Design review of the part built by this model. Coordinates are the model's own, in mm. A direction names the side the tool comes from. Round coordinates to 2 decimals unless told otherwise and drop trailing zeros. Answer as CSV lines item,"result". Start each with the question number.
(1) For faces 5 (the flat face through (10, 2.5, 27)), 6 (the cylindrical face through (-46.91, 1.52, 23.8)), list the 3-axis set-ups (+Z, -Z, +X, -X, +Y, -Y) from which the entire face can be reached by the end or side of a thin tool; tool diameter is ignored.
(2) Wall thickness on L1, parallel to Y at x = 27.5, z = -1.5: over which ranges is the line inside the solid? List them lowest first.
(3) For P1, Ø4, axis at x = 19.5, z = -27.5, coming from the +Y side, flat-tipped, find the tip position at first contact; note if it passes through.
(4) Mouldability with a two-part tool opening along X and no side actions: class faces 1 (the flat face through (20, 0, -2)), 2 (the flat face through (-54.385, 1, -1)), 3 (the flat face through (23, 2.5, -28)), 4 (the flat face through (37, 2.5, -3)) as released by +X, released by -X, zero draft, split by the parting line, or undercut.
from build123d import *

# Parameters (mm, degrees)
SKETCH1_W           = 150
SKETCH1_H           = 60
BOSS_EXTRUDE1_DEPTH = 3
CUT_EXTRUDE1_REACH  = 102.604
SKETCH2_R           = 1.75
CUT_EXTRUDE2_DEPTH  = 0.5


with BuildPart() as part:
    # Sketch1 → Boss-Extrude1 (new body)
    with BuildSketch(Plane(origin=(0, 0, 0), x_dir=(1, 0, 0), z_dir=(0, 1, 0))):
        with Locations((20.614523463, 1.144067797)):
            Rectangle(SKETCH1_W, SKETCH1_H)
    extrude(amount=BOSS_EXTRUDE1_DEPTH)

    # Sketch2 → Cut-Extrude1 (cut, up to next)
    with BuildSketch(Plane(origin=(0, 3, 0), x_dir=(1, 0, 0), z_dir=(0, 1, 0)), mode=Mode.PRIVATE) as cut_extrude1_sk1:
        with Locations(Location((-48.385476537, 25.144067797, 0), (0, 0, 270))):
            Circle(SKETCH2_R)
    cut_extrude1_tool1 = extrude(cut_extrude1_sk1.sketch, amount=-CUT_EXTRUDE1_REACH, mode=Mode.PRIVATE) & part.part
    # Sketch2 → Cut-Extrude1 (cut, up to next)
    with BuildSketch(Plane(origin=(0, 3, 0), x_dir=(1, 0, 0), z_dir=(0, 1, 0)), mode=Mode.PRIVATE) as cut_extrude1_sk2:
        with Locations(Location((-48.385476537, -22.855932203, 0), (0, 0, 270))):
            Circle(SKETCH2_R)
    cut_extrude1_tool2 = extrude(cut_extrude1_sk2.sketch, amount=-CUT_EXTRUDE1_REACH, mode=Mode.PRIVATE) & part.part
    # Sketch2 → Cut-Extrude1 (cut, up to next)
    with BuildSketch(Plane(origin=(0, 3, 0), x_dir=(1, 0, 0), z_dir=(0, 1, 0)), mode=Mode.PRIVATE) as cut_extrude1_sk3:
        with Locations(Location((89.614523463, -22.855932203, 0), (0, 0, 270))):
            Circle(SKETCH2_R)
    cut_extrude1_tool3 = extrude(cut_extrude1_sk3.sketch, amount=-CUT_EXTRUDE1_REACH, mode=Mode.PRIVATE) & part.part
    # Sketch2 → Cut-Extrude1 (cut, up to next)
    with BuildSketch(Plane(origin=(0, 3, 0), x_dir=(1, 0, 0), z_dir=(0, 1, 0)), mode=Mode.PRIVATE) as cut_extrude1_sk4:
        with Locations(Location((89.614523463, 25.144067797, 0), (0, 0, 270))):
            Circle(SKETCH2_R)
    cut_extrude1_tool4 = extrude(cut_extrude1_sk4.sketch, amount=-CUT_EXTRUDE1_REACH, mode=Mode.PRIVATE) & part.part
    add(cut_extrude1_tool1.solids().sort_by_distance((-48.385477, 3, -25.144068))[0], mode=Mode.SUBTRACT)
    add(cut_extrude1_tool2.solids().sort_by_distance((-48.385477, 3, 22.855932))[0], mode=Mode.SUBTRACT)
    add(cut_extrude1_tool3.solids().sort_by_distance((89.614523, 3, 22.855932))[0], mode=Mode.SUBTRACT)
    add(cut_extrude1_tool4.solids().sort_by_distance((89.614523, 3, -25.144068))[0], mode=Mode.SUBTRACT)

    # Sketch4 → Cut-Extrude2 (cut)
    with BuildSketch(Plane(origin=(0, 3, 0), x_dir=(1, 0, 0), z_dir=(0, 1, 0))):
        Polygon((-4.791426937, 1.38027169), (-2.904268689, -3.78923879), (2.69009548, -1.746985365), (0.802937232, 3.422525114), align=None)
        Polygon((4.072217559, 4.615993888), (17.963708333, 9.687159037), (19.814965077, 4.615993888), (5.923474302, -0.455171261), align=None)
        Polygon((0.537631953, 12.942669892), (2.424790201, 7.773159413), (8.01915437, 9.815412837), (6.131996122, 14.984923317), align=None)
        Polygon((6.855118637, 25.534649861), (8.742276884, 20.365139381), (14.336641053, 22.407392806), (12.449482806, 27.576903285), align=None)
        Polygon((-10.303537871, -10.596668593), (-8.222494664, -16.297289982), (-2.628130495, -14.255036558), (-4.709173702, -8.554415169), align=None)
        Polygon((22.734653732, -19.026845993), (24.621811979, -24.196356472), (30.216176149, -22.154103048), (28.329017901, -16.984592568), align=None)
        Polygon((28.15962548, -7.617265398), (30.046783727, -12.786775877), (35.641147896, -10.744522452), (33.753989649, -5.575011973), align=None)
        Polygon((33.470482261, 4.581220115), (35.357640508, -0.588290364), (40.952004677, 1.453963061), (39.06484643, 6.62347354), align=None)
        Polygon((39.033241178, 17.298759053), (40.920399425, 12.129248573), (46.514763594, 14.171501998), (44.627605347, 19.341012477), align=None)
        Polygon((44.260137656, 29.397485637), (46.147295903, 24.227975157), (51.741660072, 26.270228582), (49.854501825, 31.439739061), align=None)
        Polygon((-15.693454614, -23.238088767), (-13.806296367, -28.407599247), (-8.211932198, -26.365345822), (-10.099090445, -21.195835343), align=None)
        Polygon((-0.93033458, -7.272900817), (12.961156194, -2.201735668), (14.812412937, -7.272900817), (0.920922163, -12.344065966), align=None)
        Polygon((-6.074509675, -19.891339922), (7.816981099, -14.820174773), (9.668237843, -19.891339922), (-4.223252932, -24.962505072), align=None)
        Polygon((9.497387621, 16.409742117), (23.388878396, 21.480907266), (25.240135139, 16.409742117), (11.348644365, 11.338576968), align=None)
        Polygon((15.029728795, 28.514461172), (28.921219569, 33.585626321), (30.772476312, 28.514461172), (16.880985538, 23.443296023), align=None)
        Polygon((-10.862556564, -32.312872197), (3.028934211, -27.241707048), (4.880190954, -32.312872197), (-9.011299821, -37.384037346), align=None)
        Polygon((16.161463862, -27.241707048), (21.421250331, -25.321593054), (16.161463862, -10.913410108), (10.901677392, -12.833524103), align=None)
        Polygon((11.452927675, -40.137517662), (16.712714145, -38.217403668), (11.452927675, -23.809220723), (6.193141206, -25.729334717), align=None)
        Polygon((21.432742799, -15.374475147), (26.692529268, -13.454361153), (21.432742799, 0.953821792), (16.172956329, -0.966292202), align=None)
        Polygon((26.748696994, -3.629622604), (32.008483463, -1.70950861), (26.748696994, 12.698674336), (21.488910524, 10.778560341), align=None)
        Polygon((32.423035231, 8.232679073), (37.6828217, 10.152793068), (32.423035231, 24.560976013), (27.163248761, 22.640862019), align=None)
        Polygon((37.754362659, 20.558284805), (43.014149128, 22.4783988), (37.754362659, 36.886581745), (32.494576189, 34.966467751), align=None)
    extrude(amount=-CUT_EXTRUDE2_DEPTH, mode=Mode.SUBTRACT)


solid = part.part
Determined:
1,face 5,"+Y"
1,face 6,"+Y, -Y"
2,L1,"y = 0 to 2.5"
3,P1,"stops at y = 2.5"
4,face 1,"zero draft"
4,face 2,"released by -X"
4,face 3,"undercut"
4,face 4,"undercut"
